Check sheet for the modelled part. Datum: model origin and axes. Units: mm. A direction names the side the tool comes from. Give positions to 0.01 mm unless a question says otherwise; leave off trailing zeros. Write each loop counter-clockwise with the first axis right and the second up, starting at its lowest first coordinate (ties: lowest second). Pieces come first, ordered by that corner, then holes. Notation, with made-up numbers: (25.25, -18) -> (84.25, -18) arc R11 cw to (84.25, -3) -> close; hole circle Ø9 at (58.5, 38). An arc over 180 degrees is marked (long way). Use a Markdown table: item, result. Add a question column.
1. Scan lines: probe 1 along X at (y, z) = (3.75, 15.5); probe 2 along X at (y, z) = (7.95, 0); probe 3 along Z at (x, y) = (-14.5, 3). Record each from-to range of solid material in increasing order. Write a range as [from, to].
2. Cross-section at C-C (y = 28). Enter the section's corners in (x, z).
3. Gauge pin test, flat ends, axial feed: P1, Ø3, axis at x = 4.5, z = 13, coming from the +Y side; P2, Ø4, axis at x = -15.5, z = -15.5, coming from the +Y side; P3, Ø1.8, axis at x = 15.5, z = 15.5, coming from the +Y side; P4, Ø1.5, axis at y = 22.5, z = 0.5, coming from the +X side. Record the tip position at first contact, or that the pin passes through.
4. Release check for a two-part mould opening along Z. For faces 1 (the flat face through (18.2, 3.9, -18.3)), 2 (the cylindrical face through (-10.74, 9.59, -2.38)), 3 (the cylindrical face through (15.57, 3.94, 17)) record: released by +Z, released by -Z, zero draft, split by the parting line, or undercut.
5. Cross-section at B-B (x = 0). Enter the section's corners in (y, z), then the cut area to 3 significant figures.
6. Cross-section at D-D (z = -6). Enter the section's corners in (x, y), then the cut area to 3 significant figures.
7. Cross-section at A-A (z = 0). Enter the section's corners in (x, y), then the cut area to 3 significant figures.
8. Set-up check for faces 4 (the cylindrical face through (15.43, 3.94, -17)), 5 (the flat face through (2, 22, 0)), 6 (the cylindrical face through (-3.417, 9.586, -0.759)): record each of +Z, -Z, +X, -X, +Y, -Y from which the full face is reachable in a straight line by a thin tool's end or side.
from build123d import *

# Parameters (mm, degrees)
SKETCH1_W           = 42
SKETCH1_H           = 42
NEMA_17_DEPTH       = 8
CHAMFER1_SIZE       = 5.5
SKETCH2_R           = 1.5
M6_BOLT_HOLES_DEPTH = 31.757112998
SKETCH3_R           = 16
CUT_EXTRUDE1_DEPTH  = 0.2
SKETCH4_R           = 11.25
BOSS_EXTRUDE1_DEPTH = 0.8
SKETCH5_R           = 11
BOSS_EXTRUDE2_DEPTH = 2
SKETCH6_R           = 3.5
CUT_EXTRUDE2_DEPTH  = 31.918602814
SKETCH7_R           = 2.5
BOSS_EXTRUDE3_DEPTH = 24
CUT_EXTRUDE3_START  = -20
CUT_EXTRUDE3_DEPTH  = 20


with BuildPart() as part:
    # Sketch1 → Nema 17 (new body)
    with BuildSketch(Plane(origin=(0, 0, 0), x_dir=(1, 0, 0), z_dir=(0, 1, 0))):
        Rectangle(SKETCH1_W, SKETCH1_H)
    extrude(amount=NEMA_17_DEPTH)

    # Chamfer1
    chamfer1_edges = [part.edges().sort_by_distance(p)[0] for p in [
        (21, 4, 21),
        (-21, 4, 21),
        (-21, 4, -21),
        (21, 4, -21),
    ]]
    chamfer(chamfer1_edges, length=CHAMFER1_SIZE)

    # Sketch2 → M6 Bolt Holes (cut, through all)
    with BuildSketch(Plane.XZ):
        with Locations(Location((-15.5, -15.5, 0), (0, 0, 270))):
            Circle(SKETCH2_R)
        with Locations(Location((15.5, -15.5, 0), (0, 0, 90))):
            Circle(SKETCH2_R)
        with Locations(Location((-15.5, 15.5, 0), (0, 0, 90))):
            Circle(SKETCH2_R)
        with Locations(Location((15.5, 15.5, 0), (0, 0, 270))):
            Circle(SKETCH2_R)
    extrude(amount=-M6_BOLT_HOLES_DEPTH, mode=Mode.SUBTRACT)

    # Sketch3 → Cut-Extrude1 (cut)
    with BuildSketch(Plane(origin=(0, 8, 0), x_dir=(1, 0, 0), z_dir=(0, 1, 0))):
        with Locations(Location((0, 0, 0), (0, 0, 270))):
            Circle(SKETCH3_R)
    extrude(amount=-CUT_EXTRUDE1_DEPTH, mode=Mode.SUBTRACT)

    # Sketch4 → Boss-Extrude1 (add)
    with BuildSketch(Plane(origin=(0, 7.8, 0), x_dir=(1, 0, 0), z_dir=(0, 1, 0))):
        with Locations(Location((0, 0, 0), (0, 0, 270))):
            Circle(SKETCH4_R)
    extrude(amount=BOSS_EXTRUDE1_DEPTH)

    # Sketch5 → Boss-Extrude2 (add)
    with BuildSketch(Plane(origin=(0, 8.6, 0), x_dir=(1, 0, 0), z_dir=(0, 1, 0))):
        with Locations(Location((0, 0, 0), (0, 0, 270))):
            Circle(SKETCH5_R)
    extrude(amount=BOSS_EXTRUDE2_DEPTH)

    # Sketch6 → Cut-Extrude2 (cut, through all)
    with BuildSketch(Plane(origin=(0, 8.6, 0), x_dir=(1, 0, 0), z_dir=(0, 1, 0))):
        with Locations(Location((0, 0, 0), (0, 0, 270))):
            Circle(SKETCH6_R)
    extrude(amount=CUT_EXTRUDE2_DEPTH, mode=Mode.SUBTRACT)

    # Sketch7 → Boss-Extrude3 (add)
    with BuildSketch(Plane(origin=(0, 8.6, 0), x_dir=(1, 0, 0), z_dir=(0, 1, 0))):
        with Locations(Location((0, 0, 0), (0, 0, 270))):
            Circle(SKETCH7_R)
    extrude(amount=BOSS_EXTRUDE3_DEPTH)

    # Sketch9 → Cut-Extrude3 (cut)
    with BuildSketch(Plane(origin=(0, 32.6, 0), x_dir=(1, 0, 0), z_dir=(0, 1, 0)).offset(CUT_EXTRUDE3_START)):
        with BuildLine():
            Line((2, 1.5), (2, -1.5))
            ThreePointArc((2, -1.5), (2.5, 0), (2, 1.5))
        make_face()
    extrude(amount=CUT_EXTRUDE3_DEPTH, mode=Mode.SUBTRACT)


solid = part.part
Worked answers:
| question | item | result |
|---|---|---|
| 1 | probe 1 | x = [-21, -17], [-14, 14], [17, 21] |
| 1 | probe 2 | x = [-21, -16], [-11.25, 11.25], [16, 21] |
| 1 | probe 3 | z = [-21, -16.62], [-14.38, 14.38], [16.62, 21] |
| 2 | outline | (2, -1.5) -> (2, 1.5) arc R2.5 ccw (long way) to start |
| 3 | P1 | stops at y = 7.8 |
| 3 | P2 | stops at y = 8 |
| 3 | P3 | passes through |
| 3 | P4 | stops at x = 2 |
| 4 | face 1 | released by -Z |
| 4 | face 2 | split by the parting line |
| 4 | face 3 | undercut |
| 5 | outline | (0, -21) -> (8, -21) -> (8, -16) -> (7.8, -16) -> (7.8, -11.25) -> (8.6, -11.25) -> (8.6, -11) -> (10.6, -11) -> (10.6, -3.5) -> (8.6, -3.5) -> (8.6, -2.5) -> (32.6, -2.5) -> (32.6, 2.5) -> (8.6, 2.5) -> (8.6, 3.5) -> (10.6, 3.5) -> (10.6, 11) -> (8.6, 11) -> (8.6, 11.25) -> (7.8, 11.25) -> (7.8, 16) -> (8, 16) -> (8, 21) -> (0, 21) -> close |
| 5 | area | 498 mm² |
| 6 | outline | (-21, 0) -> (21, 0) -> (21, 8) -> (14.83, 8) -> (14.83, 7.8) -> (9.52, 7.8) -> (9.52, 8.6) -> (9.22, 8.6) -> (9.22, 10.6) -> (-9.22, 10.6) -> (-9.22, 8.6) -> (-9.52, 8.6) -> (-9.52, 7.8) -> (-14.83, 7.8) -> (-14.83, 8) -> (-21, 8) -> close |
| 6 | area | 382 mm² |
| 7 | outline | (-21, 0) -> (21, 0) -> (21, 8) -> (16, 8) -> (16, 7.8) -> (11.25, 7.8) -> (11.25, 8.6) -> (11, 8.6) -> (11, 10.6) -> (3.5, 10.6) -> (3.5, 8.6) -> (2.5, 8.6) -> (2.5, 12.6) -> (2, 12.6) -> (2, 32.6) -> (-2.5, 32.6) -> (-2.5, 8.6) -> (-3.5, 8.6) -> (-3.5, 10.6) -> (-11, 10.6) -> (-11, 8.6) -> (-11.25, 8.6) -> (-11.25, 7.8) -> (-16, 7.8) -> (-16, 8) -> (-21, 8) -> close |
| 7 | area | 488 mm² |
| 8 | face 4 | +Y, -Y |
| 8 | face 5 | +Z, -Z, +X, +Y |
| 8 | face 6 | +Y |
